Could you check a few things on this model? Use its own coordinates, in mm. A direction names the side the tool comes from. Give positions to 0.01 mm unless a question says otherwise; leave off trailing zeros. Write each loop counter-clockwise with the first axis right and the second up, starting at its lowest first coordinate (ties: lowest second). Pieces come first, ordered by that corner, then holes. Notation, with made-up numbers: (40, -38.75) - (65, -38.75) arc R24 cw to (65, -18.75) - close; hole circle Ø1 at (-26, 55.25). An arc over 180 degrees is marked (long way). Use one line per item in the form item = value.
```python
from build123d import *

# Parameters (mm, degrees)
F0_R     = 50
F1_DEPTH = 30
F2_SIZE  = 5


with BuildPart() as f1:
    # F0 (on Top) → F1 (new body)
    with BuildSketch(Plane.XY):
        Circle(F0_R)
        with BuildLine():
            ThreePointArc((5, 8.660254), (0, -10), (-5, 8.660254))
            Line((-5, 8.660254), (-5, 13))
            Line((-5, 13), (0, 13))
            Line((0, 13), (5, 13))
            Line((5, 13), (5, 8.660254))
        make_face(mode=Mode.SUBTRACT)
    extrude(amount=F1_DEPTH)

    # F2
    f2_edges = [f1.edges().sort_by_distance(p)[0] for p in [
        (-50, 0, 30),
        (-50, 0, 0),
    ]]
    chamfer(f2_edges, length=F2_SIZE)


solid = f1.part
```
1. Imagine slicing it at D-D, the plane z = 15.75. List the corners of the cut face in (x, y) for me, and give its area (3 significant figures).
Response values:
outline = circle Ø100 at (0, 0); hole (-5, 8.66) arc R10 ccw (long way) to (5, 8.66) - (5, 13) - (-5, 13) - close
area = 7,510 mm²
2. For pin 1 (10 mm diameter, centred on x = 3, z = 25, fed in from +Y); pin 2 (2 mm diameter, centred on y = 11.5, z = 10.5, fed in from +X); pin 3 (10 mm diameter, centred on x = 16, z = 20.5, fed in from +Y) (3 decimals), each with a flat end and sliding along its axis, tell me the tip position at first contact or that it passes through.
Response values:
pin_1 = 50
pin_2 = 48.89
pin_3 = 48.775
3. Imagine slicing it at B-B, the plane x = 0. List the corners of the cut face in (y, z) for me.
Response values:
outline = (-50, 5) - (-45, 0) - (-10, 0) - (-10, 30) - (-45, 30) - (-50, 25) - close; (13, 0) - (45, 0) - (50, 5) - (50, 25) - (45, 30) - (13, 30) - close
4. Which directions (+Z, -Z, +X, -X, +Y, -Y) give clear straight access to the entire face, cutting with the end or side of a thin tool? Please do faces 1 (the face through (41.79, -17.33, 29.76)), 2 (the face through (-5, 11, 15)).
Response values:
face_1 = +Z
face_2 = +Z, -Z
5. If I drill on line 1 (Y direction, x = 0, z = 6.75); line 2 (X direction, y = 11.5, z = 21.25); line 3 (Y direction, x = 4, z = 13), over which ranges is the centre line in solid material (lowest first)? Write a range as from..to.
Response values:
line_1 = -50..-10, 13..50
line_2 = -48.66..-5, 5..48.66
line_3 = -49.84..-9.17, 13..49.84
6. If we mould it in two halves opening along X, with no side actions, what happens to faces 3 (the face through (-11, 1, 30)), 4 (the face through (41.79, -17.33, 0.24)), 5 (the face through (0, 13, 15))? For each: pulls with the +X half, pulls with the -X half, needs draft (parallel to the pull), parting line crosses it, or undercut.
Response values:
face_3 = needs draft
face_4 = parting line crosses it
face_5 = undercut
7. Imagine slicing it at A-A, the plane y = 0. List the corners of the cut face in (x, z) for me.
Response values:
outline = (-50, 5) - (-45, 0) - (-10, 0) - (-10, 30) - (-45, 30) - (-50, 25) - close; (10, 0) - (45, 0) - (50, 5) - (50, 25) - (45, 30) - (10, 30) - close
8. Imagine slicing it at C-C, the plane z = 27. List the corners of the cut face in (x, y) for me, and give its area (3 significant figures).
Response values:
outline = circle Ø96 at (0, 0); hole (-5, 8.66) arc R10 ccw (long way) to (5, 8.66) - (5, 13) - (-5, 13) - close
area = 6,890 mm²
